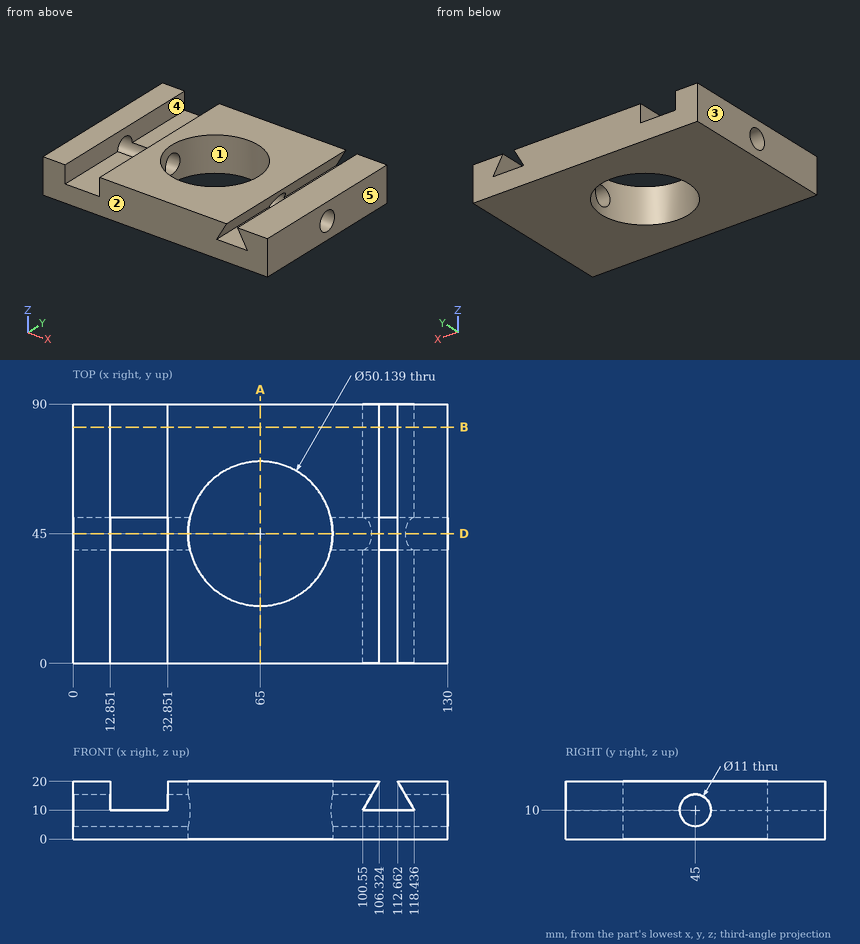
Can you work these out from the drawing? Everything is in mm from the part's minimum corner. A direction names the side the tool comes from. Give positions to 0.01 mm unless a question says otherwise; leave off trailing zeros. Loops run counter-clockwise (first coordinate to the right, second up) from the corner with the lowest first, then second, coordinate; pieces in that order, holes last. Notation, with made-up numbers: (-24, 7.5) -> (24, 7.5) arc R24 cw to (24, 45.5) -> close; hole circle Ø10 at (49.25, 27.5). An arc over 180 degrees is marked (long way). Put each result on its own line as item: value.
(1) Imagine slicing it at D-D on y = 45. State how many separate pieces and enclosed holes the cut face has.
Computed:
separate pieces: 6
enclosed holes: 0
(2) Please list where these lines run through material, in increasing order: probe 1 along Y at (x, z) = (65, 15.5); probe 2 along Z at (x, y) = (117, 45); probe 3 along Z at (x, y) = (104, 57.5) (1 decimal). Write a range as [from, to].
Computed:
probe 1: [0, 19.93], [70.07, 90]
probe 2: [0, 4.5], [15.5, 20]
probe 3: [0, 10], [16, 20]
(3) For the marked faces 4 and 5, which set-ups out of +Z, -Z, +X, -X, +Y, -Y let a thin tool reach every point of the face, with its end or its side?
Computed:
face 4: +Z, +Y, -Y
face 5: +Z, -Z, +X, +Y, -Y
(4) Imagine slicing it at A-A on x = 65. Write out the boundary of the cut face in (y, z).
Computed:
outline: (0, 0) -> (19.93, 0) -> (19.93, 20) -> (0, 20) -> close; (70.07, 0) -> (90, 0) -> (90, 20) -> (70.07, 20) -> close
(5) I'm going to push a flat-ended pin straight in: pin 1 Ø10 at (x, y) = (20, 24.5) entering from +Z. Where does the tip first touch, or does it pass through?
Computed:
pin 1: z = 10
(6) Thinking about a two-plate mould opening in X: for the marked faces 1, 2 and 3, which applies, pulls with the +X half, pulls with the -X half, needs draft (parallel to the pull), parting line crosses it, or undercut?
Computed:
face 1: undercut
face 2: needs draft
face 3: pulls with the -X half
(7) Imagine slicing it at B-B on y = 82. Write out the boundary of the cut face in (x, z), plus the area to 3 significant figures.
Computed:
outline: (0, 0) -> (130, 0) -> (130, 20) -> (112.66, 20) -> (118.44, 10) -> (100.55, 10) -> (106.32, 20) -> (32.85, 20) -> (32.85, 10) -> (12.85, 10) -> (12.85, 20) -> (0, 20) -> close
area: 2,280 mm^2
